The listing builds one solid part. Answer for the finished solid, in the listing's coordinates (mm). A direction names the side the tool comes from. Coordinates: 2 decimals unless noted, no trailing zeros. Order: outer loops, then holes, each group sorted by start corner. A loop starts at its lowest first (then second) coordinate and runs counter-clockwise, first axis right, second up. Notation, with made-up numbers: (79, 49) -> (117, 49) arc R19 cw to (117, 73) -> close; hole circle Ø9 at (81.25, 37). An arc over 180 degrees is marked (long way). One line per question, with ' | ' between items.
from build123d import *

# Parameters (mm, degrees)
SKETCH1_W           = 70
SKETCH1_H           = 100
BOSS_EXTRUDE1_DEPTH = 6
SKETCH3_W           = 60
SKETCH3_H           = 10
CUT_EXTRUDE1_DEPTH  = 5
SKETCH4_W           = 58
SKETCH4_H           = 8
CUT_EXTRUDE2_DEPTH  = 1
SKETCH5_R           = 2.5
CUT_EXTRUDE3_DEPTH  = 10
SKETCH6_R           = 4
CUT_EXTRUDE4_DEPTH  = 4.5


with BuildPart() as part:
    # Sketch1 → Boss-Extrude1 (new body)
    with BuildSketch(Plane(origin=(0, 0, 0), x_dir=(1, 0, 0), z_dir=(0, 1, 0))):
        with Locations((35, 50)):
            Rectangle(SKETCH1_W, SKETCH1_H)
    extrude(amount=BOSS_EXTRUDE1_DEPTH)

    # Sketch3 → Cut-Extrude1 (cut)
    with BuildSketch(Plane.XZ):
        with Locations((35, -20)):
            Rectangle(SKETCH3_W, SKETCH3_H)
        with Locations((35, -40)):
            Rectangle(SKETCH3_W, SKETCH3_H)
        with Locations((35, -60)):
            Rectangle(SKETCH3_W, SKETCH3_H)
        with Locations((35, -80)):
            Rectangle(SKETCH3_W, SKETCH3_H)
    extrude(amount=-CUT_EXTRUDE1_DEPTH, mode=Mode.SUBTRACT)

    # Sketch4 → Cut-Extrude2 (cut)
    with BuildSketch(Plane.XZ.offset(-5)):
        with Locations((35, -20)):
            Rectangle(SKETCH4_W, SKETCH4_H)
        with Locations((35, -40)):
            Rectangle(SKETCH4_W, SKETCH4_H)
        with Locations((35, -60)):
            Rectangle(SKETCH4_W, SKETCH4_H)
        with Locations((35, -80)):
            Rectangle(SKETCH4_W, SKETCH4_H)
    extrude(amount=-CUT_EXTRUDE2_DEPTH, mode=Mode.SUBTRACT)

    # Sketch5 → Cut-Extrude3 (cut)
    with BuildSketch(Plane.XZ):
        with Locations(Location((63, -7, 0), (0, 0, 270))):
            Circle(SKETCH5_R)
        with Locations(Location((7, -7, 0), (0, 0, 270))):
            Circle(SKETCH5_R)
        with Locations(Location((63, -93, 0), (0, 0, 270))):
            Circle(SKETCH5_R)
        with Locations(Location((7, -93, 0), (0, 0, 270))):
            Circle(SKETCH5_R)
    extrude(amount=-CUT_EXTRUDE3_DEPTH, mode=Mode.SUBTRACT)

    # Sketch6 → Cut-Extrude4 (cut)
    with BuildSketch(Plane(origin=(0, 6, 0), x_dir=(1, 0, 0), z_dir=(0, 1, 0))):
        with Locations(Location((7, 93, 0), (0, 0, 270))):
            Circle(SKETCH6_R)
        with Locations(Location((63, 93, 0), (0, 0, 90))):
            Circle(SKETCH6_R)
        with Locations(Location((63, 7, 0), (0, 0, 270))):
            Circle(SKETCH6_R)
        with Locations(Location((7, 7, 0), (0, 0, 90))):
            Circle(SKETCH6_R)
    extrude(amount=-CUT_EXTRUDE4_DEPTH, mode=Mode.SUBTRACT)


solid = part.part
Item 1: Section A-A, the plane z = -93 is taken. Give the vertices of the cut face in (x, y).
Computed values:
outline: (0, 0) -> (4.5, 0) -> (4.5, 1.5) -> (3, 1.5) -> (3, 6) -> (0, 6) -> close; (9.5, 0) -> (60.5, 0) -> (60.5, 1.5) -> (59, 1.5) -> (59, 6) -> (11, 6) -> (11, 1.5) -> (9.5, 1.5) -> close; (65.5, 0) -> (70, 0) -> (70, 6) -> (67, 6) -> (67, 1.5) -> (65.5, 1.5) -> close
Item 2: Find the intervals of material crossed by L1, parallel to Z at x = 14.5, y = 4.75; L2, parallel to X at y = 1.25, z = -93; L3, parallel to Z at x = 15, y = 5.05, in increasing order.
Computed values:
L1: z = -100 to -85, -75 to -65, -55 to -45, -35 to -25, -15 to 0 | L2: x = 0 to 4.5, 9.5 to 60.5, 65.5 to 70 | L3: z = -100 to -84, -76 to -64, -56 to -44, -36 to -24, -16 to 0
Item 3: Section B-B, the plane x = 26 is taken. Count the separate pieces of the cut face and the enclosed holes in it, plus the area to 3 significant figures.
Computed values:
separate pieces: 5 | enclosed holes: 0 | area: 368 mm^2
Item 4: For faces 1 (the face through (65, 1.5, -91)), 2 (the face through (35, 0, -51)), 3 (the face through (65, 2, -40)), determine the directions among +Z, -Z, +X, -X, +Y, -Y from which every point of the face is accessible in a straight line to the end or side of a thin tool.
Computed values:
face 1: +Y | face 2: +Z, -Z, +X, -X, -Y | face 3: -Y
Item 5: Each of these flat-tipped pins is pushed along its axis until it touches: pin 1 Ø4 at (x, z) = (7.5, -91.5) entering from +Y; pin 2 Ø3 at (x, z) = (46, -63) entering from -Y. Where does it stop, or does it pass through?
Computed values:
pin 1: stops at y = 1.5 | pin 2: stops at y = 5
